CAD build for the part. Positions are in the model's coordinates, mm. Round coordinates to 2 decimals unless told otherwise and drop trailing zeros. Write each loop counter-clockwise with the first axis right and the second up, starting at its lowest first coordinate (ties: lowest second). Pieces come first, ordered by that corner, then holes. Notation, with made-up numbers: (79, 8) - (89, 8) arc R25 cw to (89, 21) - close; hole circle Ø1 at (33, -16). An arc over 180 degrees is marked (long way). Answer in a Markdown table with one row per item.
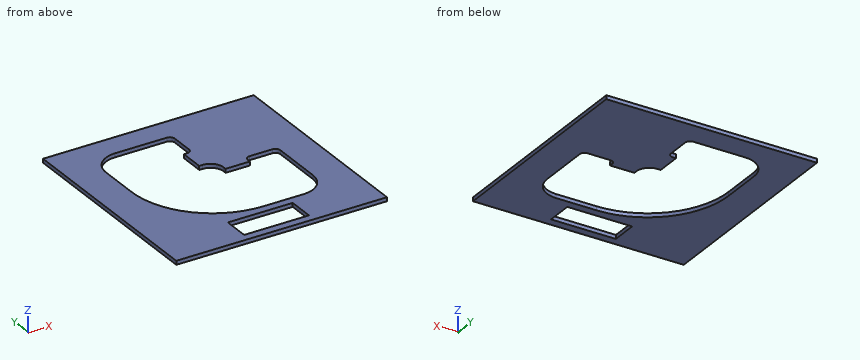
```python
from build123d import *

# Parameters (mm, degrees)
BOSS_EXTRUDE1_DEPTH = 0.12
FILLET2_R           = 1.5
FILLET3_R           = 5
BOSS_EXTRUDE2_DEPTH = 0.12
SKETCH5_W           = 1
SKETCH5_H           = 13.1
SKETCH5_W_2         = 2.922992305
SKETCH5_H_2         = 2.818599723
BOSS_EXTRUDE3_DEPTH = 0.12
FILLET5_R           = 0.3
FILLET6_R           = 0.8


with BuildPart() as part:
    # Sketch1 → Boss-Extrude1 (new, symmetric)
    with BuildSketch(Plane.XY):
        Polygon((0, 0), (-11, 0), (-11, 10.5), (-11, 11), (0, 11), (0, 10.5), align=None)
        Polygon((-1, 0.5), (-1, 5.5), (-3, 5.5), (-3, 5), (-4.5, 5), (-4.5, 6), (-5.5, 6), (-5.5, 7.5), (-5, 7.5), (-5, 9.5), (-10, 9.5), (-10, 0.5), align=None, mode=Mode.SUBTRACT)
    extrude(amount=BOSS_EXTRUDE1_DEPTH, both=True)

    # Fillet2
    fillet2_edges = [part.edges().sort_by_distance(p)[0] for p in [
        (-1, 0.5, 0),
        (-10, 9.5, 0),
    ]]
    fillet(fillet2_edges, radius=FILLET2_R)

    # Fillet3
    fillet3_edges = [part.edges().sort_by_distance(p)[0] for p in [
        (-10, 0.5, 0),
    ]]
    fillet(fillet3_edges, radius=FILLET3_R)

    # Sketch4 → Boss-Extrude2 (add, symmetric)
    with BuildSketch(Plane.XY):
        Polygon((0, 0), (0, -2.1), (-11, -2.1), (-11, 0), (-7.5, 0), (-7.5, -1.6), (-3.5, -1.6), (-3.5, 0), align=None)
    extrude(amount=BOSS_EXTRUDE2_DEPTH, both=True)

    # Sketch5 → Boss-Extrude3 (add, symmetric)
    with BuildSketch(Plane.XY):
        with Locations((-11.5, 4.45)):
            Rectangle(SKETCH5_W, SKETCH5_H)
        with Locations((0.5, 4.45)):
            Rectangle(SKETCH5_W, SKETCH5_H)
        with Locations((-1.978875572, 8.357232245)):
            Rectangle(SKETCH5_W_2, SKETCH5_H_2)
    extrude(amount=BOSS_EXTRUDE3_DEPTH, both=True)

    # Fillet5
    fillet5_edges = [part.edges().sort_by_distance(p)[0] for p in [
        (-1, 5.5, 0),
        (-3, 5.5, 0),
        (-5, 7.5, 0),
        (-5, 9.5, 0),
    ]]
    fillet(fillet5_edges, radius=FILLET5_R)

    # Fillet6
    fillet6_edges = [part.edges().sort_by_distance(p)[0] for p in [
        (-4.5, 6, 0),
    ]]
    fillet(fillet6_edges, radius=FILLET6_R)


solid = part.part
```
Q1. Drill centre lines: line 1 (Y direction, x = -2.5, z = 0); line 2 (X direction, y = 7.75, z = 0); line 3 (X direction, y = 7, z = -0.05). Where is each one in solid material? Low to high.
Computed:
| item | result |
|---|---|
| line 1 | y = -2.1 to 0.5, 5.5 to 11 |
| line 2 | x = -12 to -10, -5 to 1 |
| line 3 | x = -12 to -10, -5.5 to 1 |
Q2. Saw through at C-C on y = -0.25. List the corners of the cut face in (x, z).
Computed:
| item | result |
|---|---|
| outline | (-12, -0.12) - (-7.5, -0.12) - (-7.5, 0.12) - (-12, 0.12) - close; (-3.5, -0.12) - (1, -0.12) - (1, 0.12) - (-3.5, 0.12) - close |
Q3. Flat gauge pin, fed straight in: pin 1 (5 mm diameter, centred on x = -8, y = 7, fed in from +Z). Where does the tip first touch, or does it go through?
Computed:
| item | result |
|---|---|
| pin 1 | stops at z = 0.12 |
Q4. Saw through at B-B on z = 0.05. List the corners of the cut face in (x, y), then the cut area to 3 significant figures.
Computed:
| item | result |
|---|---|
| outline | (-12, -2.1) - (1, -2.1) - (1, 11) - (-12, 11) - close; hole (-10, 5.5) arc R5 ccw to (-5, 0.5) - (-2.5, 0.5) arc R1.5 ccw to (-1, 2) - (-1, 5.2) arc R0.3 ccw to (-1.3, 5.5) - (-2.7, 5.5) arc R0.3 ccw to (-3, 5.2) - (-3, 5) - (-4.5, 5) - (-4.5, 5.2) arc R0.8 ccw to (-5.3, 6) - (-5.5, 6) - (-5.5, 7.5) - (-5.3, 7.5) arc R0.3 ccw to (-5, 7.8) - (-5, 9.2) arc R0.3 ccw to (-5.3, 9.5) - (-8.5, 9.5) arc R1.5 ccw to (-10, 8) - close; hole (-7.5, -1.6) - (-3.5, -1.6) - (-3.5, 0) - (-7.5, 0) - close |
| area | 107 mm2 |
Q5. Saw through at A-A on x = -3.25. List the corners of the cut face in (y, z), then the cut area to 3 significant figures.
Computed:
| item | result |
|---|---|
| outline | (-2.1, -0.12) - (0.5, -0.12) - (0.5, 0.12) - (-2.1, 0.12) - close; (5, -0.12) - (11, -0.12) - (11, 0.12) - (5, 0.12) - close |
| area | 2.06 mm2 |
